Work out the finished part from the listing and answer in its coordinate system (mm). A direction names the side the tool comes from. Round coordinates to 2 decimals unless told otherwise and drop trailing zeros. Order: outer loops, then holes, each group sorted by start corner. A loop starts at its lowest first (then second) coordinate and runs counter-clockwise, first axis right, second up. Notation, with made-up numbers: M 62.5,37.5 L 75.5,37.5 A10 ccw 75.5,52.5 Z; hole C 75,11.5 d4. An arc over 180 degrees is marked long. Return JSON: item names as keys, results as strings.
from build123d import *

# Parameters (mm, degrees)
SKETCH1_W           = 40
SKETCH1_H           = 40
BOSS_EXTRUDE1_DEPTH = 6
SKETCH2_W           = 40
SKETCH2_H           = 40
SKETCH2_R           = 4.5
BOSS_EXTRUDE2_DEPTH = 3
SKETCH3_R           = 2.5
CUT_EXTRUDE1_DEPTH  = 24
SKETCH4_R           = 7.5
SKETCH4_R_2         = 4.5
BOSS_EXTRUDE3_DEPTH = 7
FILLET1_R           = 3


with BuildPart() as part:
    # Sketch1 → Boss-Extrude1 (new body)
    with BuildSketch(Plane(origin=(0, 0, 0), x_dir=(1, 0, 0), z_dir=(0, 1, 0))):
        Rectangle(SKETCH1_W, SKETCH1_H)
        Polygon((7.505553499, 0), (3.75277675, 6.5), (-3.75277675, 6.5), (-7.505553499, 0), (-3.75277675, -6.5), (3.75277675, -6.5), align=None, mode=Mode.SUBTRACT)
    extrude(amount=BOSS_EXTRUDE1_DEPTH)

    # Sketch2 → Boss-Extrude2 (add)
    with BuildSketch(Plane(origin=(0, 6, 0), x_dir=(1, 0, 0), z_dir=(0, 1, 0))):
        Rectangle(SKETCH2_W, SKETCH2_H)
        with Locations(Location((0, 0, 0), (0, 0, 270))):
            Circle(SKETCH2_R, mode=Mode.SUBTRACT)
    extrude(amount=BOSS_EXTRUDE2_DEPTH)

    # Sketch3 → Cut-Extrude1 (cut)
    with BuildSketch(Plane(origin=(0, 9, 0), x_dir=(1, 0, 0), z_dir=(0, 1, 0))):
        with Locations(Location((-11.514718626, 11.514718626, 0), (0, 0, 270))):
            Circle(SKETCH3_R)
        with Locations(Location((11.514718626, 11.514718626, 0), (0, 0, 270))):
            Circle(SKETCH3_R)
        with Locations(Location((11.514718626, -11.514718626, 0), (0, 0, 270))):
            Circle(SKETCH3_R)
        with Locations(Location((-11.514718626, -11.514718626, 0), (0, 0, 270))):
            Circle(SKETCH3_R)
    extrude(amount=-CUT_EXTRUDE1_DEPTH, mode=Mode.SUBTRACT)

    # Sketch4 → Boss-Extrude3 (add)
    with BuildSketch(Plane(origin=(0, 9, 0), x_dir=(1, 0, 0), z_dir=(0, 1, 0))):
        with Locations(Location((0, 0, 0), (0, 0, 90))):
            Circle(SKETCH4_R)
        with Locations(Location((0, 0, 0), (0, 0, 270))):
            Circle(SKETCH4_R_2, mode=Mode.SUBTRACT)
    extrude(amount=BOSS_EXTRUDE3_DEPTH)

    # Fillet1
    fillet1_edges = [part.edges().sort_by_distance(p)[0] for p in [
        (0, 9, 7.5),
    ]]
    fillet(fillet1_edges, radius=FILLET1_R)


solid = part.part
Item 1: Consider line 1 along Z through (x, y) = (-11.5, 8.25); line 2 along Z through (x, y) = (2.5, 7.75); line 3 along X through (y, z) = (8.5, 0). Determine where each line is inside the solid, lowest interval first. Write a range as [from, to].
Output:
{"line 1": "z = [-20, -14.01], [-9.01, 9.01], [14.01, 20]", "line 2": "z = [-20, -3.74], [3.74, 20]", "line 3": "x = [-20, -4.5], [4.5, 20]"}
Item 2: Each of these flat-tipped pins is pushed along its axis until it touches: pin 1 (12 mm diameter, centred on x = -10.5, z = -5, fed in from +Y); pin 2 (1 mm diameter, centred on x = 1, y = 12.5, fed in from -Z); pin 3 (4.5 mm diameter, centred on x = 11.51, z = -11.51, fed in from -Y); pin 4 (8 mm diameter, centred on x = 11.51, z = 11.51, fed in from +Y). Where does it stop, or does it pass through?
Output:
{"pin 1": "stops at y = 16", "pin 2": "stops at z = -7.48", "pin 3": "passes through", "pin 4": "stops at y = 9"}
Item 3: The mould has two halves that part along X. Classify faces 4 (the flat face through (0, 4, -20)), 5 (the flat face through (-20, 4, 0)), 6 (the cylindrical face through (-13.036, 4.563, 9.531)): pulls with the +X half, pulls with the -X half, needs draft (parallel to the pull), parting line crosses it, or undercut.
Output:
{"face 4": "needs draft", "face 5": "pulls with the -X half", "face 6": "undercut"}
Item 4: Which of the six approach directions +Z, -Z, +X, -X, +Y, -Y give full straight-line access (tool end or side, diameter ignored) to faces 1 (the flat face through (0, 3, 6.5)), 2 (the cylindrical face through (11.625, 4.563, -14.012)), 3 (the flat face through (-9, 9, -9))?
Output:
{"face 1": "-Y", "face 2": "+Y, -Y", "face 3": "+Y"}
Item 5: Find section B-B (x = -13.5). Determine the outline of the cut face in (y, z).
Output:
{"outline": "M 0,-20 L 9,-20 L 9,-13.03 L 0,-13.03 Z; M 0,-10 L 9,-10 L 9,10 L 0,10 Z; M 0,13.03 L 9,13.03 L 9,20 L 0,20 Z"}
Item 6: Find section C-C (y = 1.5). Determine the outline of the cut face in (x, z).
Output:
{"outline": "M -20,-20 L 20,-20 L 20,20 L -20,20 Z; hole C -11.51,-11.51 d5; hole C -11.51,11.51 d5; hole M -7.51,0 L -3.75,-6.5 L 3.75,-6.5 L 7.51,0 L 3.75,6.5 L -3.75,6.5 Z; hole C 11.51,-11.51 d5; hole C 11.51,11.51 d5"}
Item 7: Find section D-D (x = 16.5). Determine the outline of the cut face in (y, z).
Output:
{"outline": "M 0,-20 L 9,-20 L 9,20 L 0,20 Z"}
Item 8: Find section A-A (x = 0). Determine the outline of the cut face in (y, z).
Output:
{"outline": "M 0,-20 L 9,-20 L 9,-10.5 A3 cw 12,-7.5 L 16,-7.5 L 16,-4.5 L 6,-4.5 L 6,-6.5 L 0,-6.5 Z; M 0,6.5 L 6,6.5 L 6,4.5 L 16,4.5 L 16,7.5 L 12,7.5 A3 cw 9,10.5 L 9,20 L 0,20 Z"}
